Answer from the drawing. Dimensions are ordinates in mm from the lowest x, y and z of the part. A direction names the side the tool comes from. Coordinates: 2 decimals unless noted, no trailing zeros.
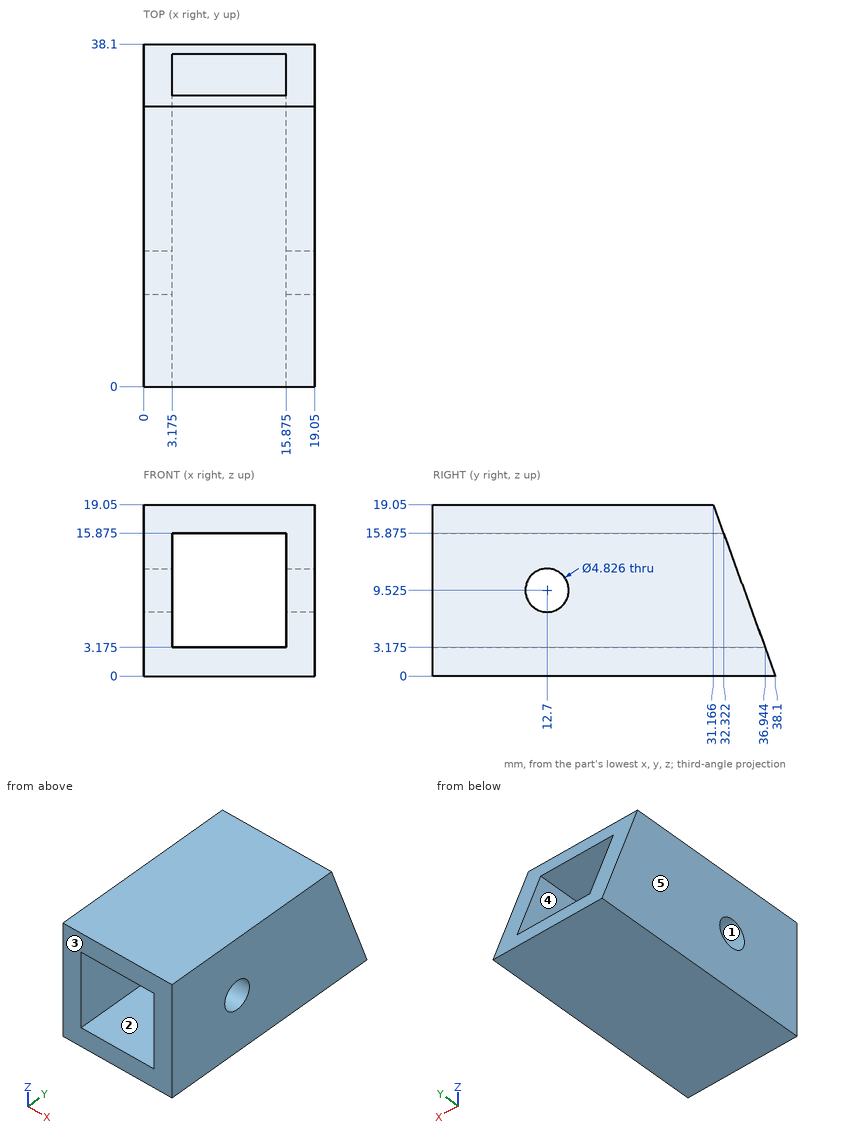
Item 1: Given pin 1 (1.5 mm diameter, centred on x = 10, y = 19, fed in from -Z); pin 2 (3 mm diameter, centred on y = 12.7, z = 9.525, fed in from +X); pin 3 (8 mm diameter, centred on x = 3.5, z = 10, fed in from +Y), each flat-ended and moving along its own axis, determine where each tip first touches the part or whether it passes through.
Numbers:
pin 1: stops at z = 0
pin 2: passes through
pin 3: stops at y = 35.91
Item 2: Find the intervals of material crossed by line 1 along Y through (x, z) = (17.5, 11.75) (1 decimal); line 2 along Z through (x, y) = (1, 13.5); line 3 along Y through (x, z) = (16.75, 16.75), in increasing order.
Numbers:
line 1: y = 0 to 11.8, 13.6 to 33.8
line 2: z = 0 to 7.25, 11.8 to 19.05
line 3: y = 0 to 32
Item 3: Determine the mould class of the marked faces 1, 2 and 3 for opening direction Y: released by +Y, released by -Y, zero draft, split by the parting line, or undercut.
Numbers:
face 1: undercut
face 2: zero draft
face 3: released by -Y
Item 4: Which of the six approach directions +Z, -Z, +X, -X, +Y, -Y give full straight-line access (tool end or side, diameter ignored) to the marked faces 4 and 5?
Numbers:
face 4: +Y, -Y
face 5: +Z, -Z, -X, +Y, -Y
